Could you check a few things on this model? Use its own coordinates, in mm. A direction names the side the tool comes from. Give positions to 0.01 mm unless a question says otherwise; leave off trailing zeros. Loops run counter-clockwise (first coordinate to the right, second up) from the corner with the lowest first, then second, coordinate; pieces in that order, holes last. Notation, with made-up numbers: (31, 66.5) - (68, 66.5) arc R27 ccw to (68, 89.5) - close; hole circle Ø9 at (39.5, -26.5). An arc over 180 degrees is marked (long way). One line per item, written item: value. Start each with the question number.
Q1. I want a section at B-B (y = 0). Please give me the cut outline in (x, z).
Q2. If I drill on line 1 (Y direction, x = 8, z = -2.7); line 2 (X direction, y = -6, z = -2.4); line 3 (Y direction, x = -1, z = -3.2), over which ranges is the centre line in solid material (lowest first)? Write a range as from..to.
Q3. If we mould it in two halves opening along Y, with no side actions, what happens to faces 3 (the face through (0, -7.5, -2)), 4 (the face through (0, -9.5, -2)), 5 (the face through (0, 9.5, -2)), 6 (the face through (17, 0, -2))? For each: released by +Y, released by -Y, zero draft, split by the parting line, or undercut.
Q4. I want a section at A-A (x = 8). Please give me the cut outline in (y, z).
Q5. I want a section at C-C (x = -10.5). Please give me the cut outline in (y, z), then the cut area to 3 significant figures.
Q6. For faces 1 (the face through (-11, -5, -2)), 2 (the face through (0, 0, 0)), which set-ups out of +Z, -Z, +X, -X, +Y, -Y let a thin tool reach every point of the face, with its end or its side?
Q7. I want a section at D-D (z = -3.3). Please give me the cut outline in (x, y), then the cut area to 3 significant figures.
```python
from build123d import *

# Parameters (mm, degrees)
F0_W     = 22
F0_H     = 5
F0_R     = 2
F1_DEPTH = 5
F3_D     = 4
F4_DEPTH = 5
F6_D     = 3


with BuildPart() as f1:
    # F0 (on Top) → F1 (new body)
    with BuildSketch(Plane.XY):
        Polygon((17, 0), (17, 9.5), (-17, 9.5), (-17, 0), (-17, -7.5), (-17, -9.5), (-11, -9.5), (14, -9.5), (17, -9.5), (17, -7.5), align=None)
        with Locations((0, -5)):
            Rectangle(F0_W, F0_H, mode=Mode.SUBTRACT)
        with BuildLine():
            ThreePointArc((-12, 0), (-14, -2), (-16, 0))
            ThreePointArc((-16, 0), (-14, 2), (-12, 0))
        make_face(mode=Mode.SUBTRACT)
        with Locations((14, 0)):
            Circle(F0_R, mode=Mode.SUBTRACT)
    extrude(amount=-F1_DEPTH)

    # F3 (through all)
    with Locations(Plane.XY):
        with Locations((13, 0)):
            Hole(F3_D / 2)

    # F0 (on Top) → F4 (join)
    with BuildSketch(Plane.XY):
        with BuildLine():
            ThreePointArc((-12, 0), (-14, 2), (-16, 0))
            ThreePointArc((-16, 0), (-14, -2), (-12, 0))
        make_face()
        with Locations((14, 0)):
            Circle(F0_R)
        Polygon((17, 0), (17, 9.5), (-17, 9.5), (-17, 0), (-17, -7.5), (-17, -9.5), (-11, -9.5), (14, -9.5), (17, -9.5), (17, -7.5), align=None)
        with Locations((0, -5)):
            Rectangle(F0_W, F0_H, mode=Mode.SUBTRACT)
        with BuildLine():
            ThreePointArc((-12, 0), (-14, -2), (-16, 0))
            ThreePointArc((-16, 0), (-14, 2), (-12, 0))
        make_face(mode=Mode.SUBTRACT)
        with Locations((14, 0)):
            Circle(F0_R, mode=Mode.SUBTRACT)
    extrude(amount=-F4_DEPTH)

    # F6 (through all)
    with Locations(Plane.XY):
        with Locations((-8, 4.5), (8, 4.5)):
            Hole(F6_D / 2)


solid = f1.part
```
Worked answers:
1. outline: (-17, -5) - (-16, -5) - (-16, 0) - (-17, 0) - close; (-12, -5) - (12, -5) - (12, 0) - (-12, 0) - close; (16, -5) - (17, -5) - (17, 0) - (16, 0) - close
2. line 1: y = -9.5..-7.5, -2.5..3, 6..9.5
2. line 2: x = -17..-11, 11..17
2. line 3: y = -9.5..-7.5, -2.5..9.5
3. face 3: undercut
3. face 4: released by -Y
3. face 5: released by +Y
3. face 6: zero draft
4. outline: (-9.5, -5) - (-7.5, -5) - (-7.5, 0) - (-9.5, 0) - close; (-2.5, -5) - (3, -5) - (3, 0) - (-2.5, 0) - close; (6, -5) - (9.5, -5) - (9.5, 0) - (6, 0) - close
5. outline: (-9.5, -5) - (-7.5, -5) - (-7.5, 0) - (-9.5, 0) - close; (-2.5, -5) - (9.5, -5) - (9.5, 0) - (-2.5, 0) - close
5. area: 70.0 mm²
6. face 1: +Z, -Z
6. face 2: +Z, +X, -X, +Y, -Y
7. outline: (-17, -9.5) - (17, -9.5) - (17, 9.5) - (-17, 9.5) - close; hole circle Ø4 at (-14, 0); hole (-11, -7.5) - (11, -7.5) - (11, -2.5) - (-11, -2.5) - close; hole circle Ø3 at (-8, 4.5); hole circle Ø3 at (8, 4.5); hole circle Ø4 at (14, 0)
7. area: 497 mm²
